For this review, take the finished solid that the model builds, in its own axes (mm). A direction names the side the tool comes from. Coordinates: 2 decimals unless noted, no trailing zeros. Loops run counter-clockwise (first coordinate to the right, second up) from the corner with the lowest first, then second, coordinate; pieces in that order, holes last.
```python
from build123d import *

# Parameters (mm, degrees)
SKETCH2_W           = 600
SKETCH2_H           = 400
BOSS_EXTRUDE1_DEPTH = 600
SHELL1_T            = -50
SKETCH3_R           = 2.5
CUT_EXTRUDE1_DEPTH  = 872.779788708
SKETCH4_R           = 2.5
CUT_EXTRUDE2_DEPTH  = 275
LPATTERN1_COUNT     = 8
LPATTERN1_PITCH     = 50
SKETCH5_R           = 2.5
CUT_EXTRUDE3_DEPTH  = 872.779788708


with BuildPart() as part:
    # Sketch2 → Boss-Extrude1 (new body)
    with BuildSketch(Plane(origin=(0, 0, 0), x_dir=(1, 0, 0), z_dir=(0, 1, 0))):
        Rectangle(SKETCH2_W, SKETCH2_H)
    extrude(amount=BOSS_EXTRUDE1_DEPTH)

    # Shell1
    shell1_openings = [part.faces().sort_by_distance(p)[0] for p in [
        (0, 300, -200),
    ]]
    offset(amount=SHELL1_T, openings=shell1_openings, kind=Kind.INTERSECTION)

    # Sketch3 → Cut-Extrude1 (cut, through all)
    with BuildSketch(Plane.ZY.offset(300)):
        with Locations((-175, 100)):
            Circle(SKETCH3_R)
        with Locations((-175, 130)):
            Circle(SKETCH3_R)
        with Locations((-175, 470)):
            Circle(SKETCH3_R)
        with Locations((-175, 500)):
            Circle(SKETCH3_R)
    extrude(amount=-CUT_EXTRUDE1_DEPTH, mode=Mode.SUBTRACT)

    # Sketch4 → Cut-Extrude2 (cut, symmetric)
    with BuildSketch(Plane(origin=(0, 0, 0), x_dir=(0, 0, -1), z_dir=(1, 0, 0))):
        with Locations((-105, 130)):
            Circle(SKETCH4_R)
        with Locations((145, 130)):
            Circle(SKETCH4_R)
    cut_extrude2 = extrude(amount=CUT_EXTRUDE2_DEPTH, both=True, mode=Mode.SUBTRACT)

    # LPattern1: Cut-Extrude2 ×8
    with Locations(*[(0, i * LPATTERN1_PITCH, 0) for i in range(1, LPATTERN1_COUNT)]):
        add(cut_extrude2, mode=Mode.SUBTRACT)

    # Sketch5 → Cut-Extrude3 (cut, through all)
    with BuildSketch(Plane.ZY.offset(300)):
        with Locations((0, 20)):
            Circle(SKETCH5_R)
        with Locations((30, 20)):
            Circle(SKETCH5_R)
    extrude(amount=-CUT_EXTRUDE3_DEPTH, mode=Mode.SUBTRACT)


solid = part.part
```
Q1. Machinability: for faces 1 (the face through (250, 296, -23)), 2 (the face through (-300, 296, 3)), which of the approach directions +Z, -Z, +X, -X, +Y, -Y give a long, thin tool a straight path to every point of the face, cutting with its end or side? Answer none if there is none.
Q2. For pin 1 Ø5 at (x, y) = (-37, 370.5) entering from -Z, flat-tipped, find the tip position at first contact; note if it passes through.
Q3. Consider section A-A (z = -32.5). State the section outline as (x, y) points, then the cut area to 3 significant figures.
Q4. The part is to be moulded in two halves that separate along Y. For faces 3 (the face through (-3, 550, -27)), 4 (the face through (300, 296, 3)), 5 (the face through (-4, 0, -3)), say which applies: +Y half, -Y half, draft (parallel to the pull), parting line (faces both ways), or undercut.
Q5. Consider section B-B (x = -177). State the section outline as (y, z) points.
Q6. Wall thickness on probe 1 along Y at (x, z) = (-280, -175); probe 2 along Z at (x, y) = (258.75, 280); probe 3 along X at (y, z) = (212, 121): over which ranges is each line inside the solid? List them lowest first.
Model answer:
1. face 1: -Z
1. face 2: +Z, -Z, -X, +Y, -Y
2. pin 1: stops at z = 150
3. outline: (-300, 0) - (300, 0) - (300, 600) - (-300, 600) - close; hole (-250, 50) - (250, 50) - (250, 550) - (-250, 550) - close
3. area: 110,000 mm2
4. face 3: undercut
4. face 4: draft
4. face 5: -Y half
5. outline: (0, -200) - (50, -200) - (50, 150) - (550, 150) - (550, -200) - (600, -200) - (600, 200) - (0, 200) - close; hole circle Ø5 at (20, 0); hole circle Ø5 at (20, 30)
6. probe 1: y = 0 to 97.5, 102.5 to 127.5, 132.5 to 467.5, 472.5 to 497.5, 502.5 to 600
6. probe 2: z = -200 to -147.5, -142.5 to 102.5, 107.5 to 200
6. probe 3: x = -300 to -250, 250 to 300
